Geometry: final body of the model. Coordinates: model frame, mm. Give positions to 0.01 mm unless a question says otherwise; leave off trailing zeros. Loops run counter-clockwise (first coordinate to the right, second up) from the corner with the lowest first, then second, coordinate; pieces in that order, holes last. Notation, with made-up numbers: (78.25, 66.5) -> (124.25, 66.5) arc R34 ccw to (124.25, 97.5) -> close; hole circle Ø1 at (-11, 37). An arc over 180 degrees is marked (long way). Answer in a Markdown table with one row per item. Add a question column.
Autodesk Inventor part; units mm, degrees
ref_plane "YZ Plane" through (0, 0, 0) normal (1, 0, 0) x (0, 1, 0)
ref_plane "XZ Plane" through (0, 0, 0) normal (0, 1, 0) x (-1, 0, 0)
ref_plane "XY Plane" through (0, 0, 0) normal (0, 0, 1) x (1, 0, 0)
sketch "Sketch1" plane through (0, 0, 0) normal (0, 1, 0) x (-1, 0, 0)
  circle A0 centre (0, 0) radius 45
  dimension "d1" = 90
extrude "Extrusion1" add sketch "Sketch1" along normal blind 10
sketch "Sketch2" plane through (0, 10, 0) normal (0, 1, 0) x (1, 0, 0)
  circle A0 centre (0, 0) radius 16
  dimension "d4" = 32
hole "Hole1" at (0, 10, 0) direction (0, -1, 0) diameter 35 end through all
sketch "Sketch4" plane through (0, 10, 0) normal (0, 1, 0) x (1, 0, 0)
  point P0 (0, 0)
sketch "Sketch5" plane through (0, 10, 0) normal (0, 1, 0) x (1, 0, 0)
  circle A0 centre (-30, 0) radius 4
  circle A1 centre (-27.4064, -12.2021) radius 4
  circle A2 centre (-20.0739, -22.2943) radius 4
  circle A3 centre (-9.2705, -28.5317) radius 4
  circle A4 centre (3.1359, -29.8357) radius 4
  circle A5 centre (15, -25.9808) radius 4
  circle A6 centre (24.2705, -17.6336) radius 4
  circle A7 centre (29.3444, -6.2374) radius 4
  circle A8 centre (29.3444, 6.2374) radius 4
  circle A9 centre (24.2705, 17.6336) radius 4
  circle A10 centre (15, 25.9808) radius 4
  circle A11 centre (3.1359, 29.8357) radius 4
  circle A12 centre (-9.2705, 28.5317) radius 4
  circle A13 centre (-20.0739, 22.2943) radius 4
  circle A14 centre (-27.4064, 12.2021) radius 4
  point P0 (0, 0)
  dimension "d29" = 8
  dimension "d30" = 30
  dimension "d33" = 360
hole "Hole3" at (-27.4064, 10, 12.2021) at (-30, 10, 0) at (-27.4064, 10, -12.2021) at (-20.0739, 10, -22.2943) at (-9.2705, 10, -28.5317) at (3.1359, 10, -29.8357) at (15, 10, -25.9808) at (24.2705, 10, -17.6336) at (29.3444, 10, -6.2374) at (29.3444, 10, 6.2374) at (24.2705, 10, 17.6336) at (15, 10, 25.9808) at (3.1359, 10, 29.8357) at (-9.2705, 10, 28.5317) at (-20.0739, 10, 22.2943) direction (0, -1, 0) diameter 8 end through all
sketch "Sketch7" plane through (0, 10, 0) normal (0, 1, 0) x (1, 0, 0)
  point P0 (0, 0)
properties part number "Orifice Plate" material "Stainless Steel"
(1) Cut plane B-B on x = -30. Return the cut outline in (y, z).
(2) Material intervals for line 1 along Z through (x, y) = (-19, 8); line 2 along X through (y, z) = (2, 5); line 3 along Z through (x, y) = (30, 1.5), sorted ascending. Write a range as from..to.
(3) Draft query along Z for faces 1 (the cylindrical face through (2.96, 4.93, -33.83)), 2 (the flat face through (1, 0, -19)), 3 (the cylindrical face through (-20.765, 4.93, 39.923)). Return one class per face: +Z half, -Z half, draft (parallel to the pull), parting line (faces both ways), or undercut.
(4) Cut plane D-D on x = -2.5. Return the cut outline in (y, z).
(5) Cut plane C-C on y = 7.75. State how many separate pieces and enclosed holes the cut face has, then the cut area to 3 significant figures.
(6) Cut plane A-A on z = 0. Return the cut outline in (x, y), then the cut area to 3 significant figures.
(7) Pin query (flat end, axial travel): pin 1 Ø7 at (x, z) = (-20.07, 22.29) entering from -Y; pin 2 Ø10.5 at (x, z) = (-30, 0) entering from +Y; pin 3 Ø6 at (y, z) = (4, 20) entering from +X; pin 4 Ø5 at (y, z) = (1.5, 5.5) entering from +X. Return the tip coordinate at first contact, or that it passes through.
Answer list:
| question | item | result |
|---|---|---|
| 1 | outline | (0, -33.54) -> (10, -33.54) -> (10, -15.25) -> (0, -15.25) -> close; (0, -9.16) -> (10, -9.16) -> (10, -4) -> (0, -4) -> close; (0, 4) -> (10, 4) -> (10, 9.16) -> (0, 9.16) -> close; (0, 15.25) -> (10, 15.25) -> (10, 33.54) -> (0, 33.54) -> close |
| 2 | line 1 | z = -40.79..-26.15, -18.44..18.44, 26.15..40.79 |
| 2 | line 2 | x = -44.72..-16.77, 16.77..25.54, 33.15..44.72 |
| 2 | line 3 | z = -33.54..-10.18, -2.29..2.29, 10.18..33.54 |
| 3 | face 1 | undercut |
| 3 | face 2 | draft |
| 3 | face 3 | parting line |
| 4 | outline | (0, -44.93) -> (10, -44.93) -> (10, -17.32) -> (0, -17.32) -> close; (0, 17.32) -> (10, 17.32) -> (10, 44.93) -> (0, 44.93) -> close |
| 5 | separate pieces | 1 |
| 5 | enclosed holes | 16 |
| 5 | area | 4,650 mm² |
| 6 | outline | (-45, 0) -> (-34, 0) -> (-34, 10) -> (-45, 10) -> close; (-26, 0) -> (-17.5, 0) -> (-17.5, 10) -> (-26, 10) -> close; (17.5, 0) -> (45, 0) -> (45, 10) -> (17.5, 10) -> close |
| 6 | area | 470 mm² |
| 7 | pin 1 | passes through |
| 7 | pin 2 | stops at y = 10 |
| 7 | pin 3 | stops at x = 41.67 |
| 7 | pin 4 | stops at x = 44.9 |
